Read the model definition and answer for the solid it produces. Units are mm, in the model's axes. Round coordinates to 2 decimals unless told otherwise and drop trailing zeros. Write each loop counter-clockwise with the first axis right and the second up, starting at its lowest first coordinate (ties: lowest second). Pieces come first, ordered by that corner, then holes.
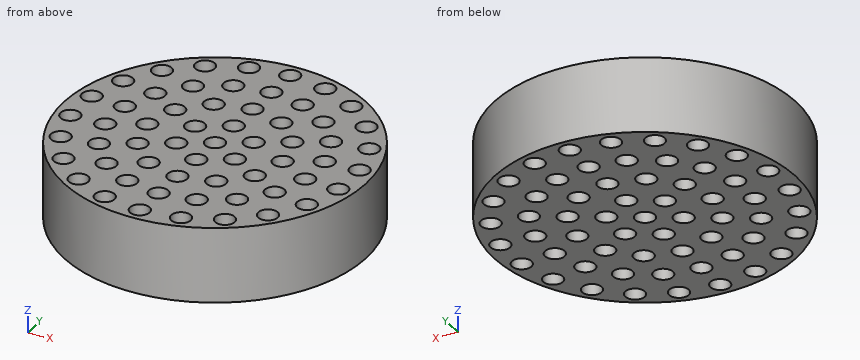
from build123d import *

# Parameters (mm, degrees)
ESQUISSE1_R             = 20
BOSS_EXTRU_1_DEPTH      = 10
ESQUISSE2_R             = 1.3
ENL_V_MAT_EXTRU_1_DEPTH = 10


with BuildPart() as part:
    # Esquisse1 → Boss.-Extru.1 (new body)
    with BuildSketch(Plane.XY):
        Circle(ESQUISSE1_R)
    extrude(amount=BOSS_EXTRU_1_DEPTH)

    # Esquisse2 → Enlèv. mat.-Extru.1 (cut)
    with BuildSketch(Plane.XY.offset(10)):
        with Locations((0, 4.5)):
            Circle(ESQUISSE2_R)
        with Locations((-3.897114317, 2.25)):
            Circle(ESQUISSE2_R)
        with Locations((-3.897114317, -2.25)):
            Circle(ESQUISSE2_R)
        with Locations((0, -4.5)):
            Circle(ESQUISSE2_R)
        with Locations((3.897114317, -2.25)):
            Circle(ESQUISSE2_R)
        with Locations((3.897114317, 2.25)):
            Circle(ESQUISSE2_R)
        Circle(ESQUISSE2_R)
        with Locations((0, 9)):
            Circle(ESQUISSE2_R)
        with Locations((4.5, 7.794228634)):
            Circle(ESQUISSE2_R)
        with Locations((7.794228634, 4.5)):
            Circle(ESQUISSE2_R)
        with Locations((9, 0)):
            Circle(ESQUISSE2_R)
        with Locations((7.794228634, -4.5)):
            Circle(ESQUISSE2_R)
        with Locations((4.5, -7.794228634)):
            Circle(ESQUISSE2_R)
        with Locations((0, -9)):
            Circle(ESQUISSE2_R)
        with Locations((-4.5, -7.794228634)):
            Circle(ESQUISSE2_R)
        with Locations((-7.794228634, -4.5)):
            Circle(ESQUISSE2_R)
        with Locations((-9, 0)):
            Circle(ESQUISSE2_R)
        with Locations((-7.794228634, 4.5)):
            Circle(ESQUISSE2_R)
        with Locations((-4.5, 7.794228634)):
            Circle(ESQUISSE2_R)
        with Locations((0, 13.5)):
            Circle(ESQUISSE2_R)
        with Locations((0, 18)):
            Circle(ESQUISSE2_R)
        with Locations((4.617271935, 12.685850381)):
            Circle(ESQUISSE2_R)
        with Locations((8.677632731, 10.341599982)):
            Circle(ESQUISSE2_R)
        with Locations((11.691342951, 6.75)):
            Circle(ESQUISSE2_R)
        with Locations((13.294904666, 2.344250399)):
            Circle(ESQUISSE2_R)
        with Locations((13.294904666, -2.344250399)):
            Circle(ESQUISSE2_R)
        with Locations((11.691342951, -6.75)):
            Circle(ESQUISSE2_R)
        with Locations((8.677632731, -10.341599982)):
            Circle(ESQUISSE2_R)
        with Locations((4.617271935, -12.685850381)):
            Circle(ESQUISSE2_R)
        with Locations((0, -13.5)):
            Circle(ESQUISSE2_R)
        with Locations((-4.617271935, -12.685850381)):
            Circle(ESQUISSE2_R)
        with Locations((-8.677632731, -10.341599982)):
            Circle(ESQUISSE2_R)
        with Locations((-11.691342951, -6.75)):
            Circle(ESQUISSE2_R)
        with Locations((-13.294904666, -2.344250399)):
            Circle(ESQUISSE2_R)
        with Locations((-13.294904666, 2.344250399)):
            Circle(ESQUISSE2_R)
        with Locations((-11.691342951, 6.75)):
            Circle(ESQUISSE2_R)
        with Locations((-8.677632731, 10.341599982)):
            Circle(ESQUISSE2_R)
        with Locations((-4.617271935, 12.685850381)):
            Circle(ESQUISSE2_R)
        with Locations((5.071186023, 17.270873525)):
            Circle(ESQUISSE2_R)
        with Locations((9.731534714, 15.142563591)):
            Circle(ESQUISSE2_R)
        with Locations((13.603492338, 11.787493211)):
            Circle(ESQUISSE2_R)
        with Locations((16.373375916, 7.477470234)):
            Circle(ESQUISSE2_R)
        with Locations((17.816785954, 2.561667089)):
            Circle(ESQUISSE2_R)
        with Locations((17.816785954, -2.561667089)):
            Circle(ESQUISSE2_R)
        with Locations((16.373375916, -7.477470234)):
            Circle(ESQUISSE2_R)
        with Locations((13.603492338, -11.787493211)):
            Circle(ESQUISSE2_R)
        with Locations((9.731534714, -15.142563591)):
            Circle(ESQUISSE2_R)
        with Locations((5.071186023, -17.270873525)):
            Circle(ESQUISSE2_R)
        with Locations((0, -18)):
            Circle(ESQUISSE2_R)
        with Locations((-5.071186023, -17.270873525)):
            Circle(ESQUISSE2_R)
        with Locations((-9.731534714, -15.142563591)):
            Circle(ESQUISSE2_R)
        with Locations((-13.603492338, -11.787493211)):
            Circle(ESQUISSE2_R)
        with Locations((-16.373375916, -7.477470234)):
            Circle(ESQUISSE2_R)
        with Locations((-17.816785954, -2.561667089)):
            Circle(ESQUISSE2_R)
        with Locations((-17.816785954, 2.561667089)):
            Circle(ESQUISSE2_R)
        with Locations((-16.373375916, 7.477470234)):
            Circle(ESQUISSE2_R)
        with Locations((-13.603492338, 11.787493211)):
            Circle(ESQUISSE2_R)
        with Locations((-9.731534714, 15.142563591)):
            Circle(ESQUISSE2_R)
        with Locations((-5.071186023, 17.270873525)):
            Circle(ESQUISSE2_R)
    extrude(amount=-ENL_V_MAT_EXTRU_1_DEPTH, mode=Mode.SUBTRACT)


solid = part.part
Q1. Section C-C (y = -18) is taken. Determine the outline of the cut face in (x, z).
Verdict:
outline: (-8.72, 0) - (-6.15, 0) - (-6.15, 10) - (-8.72, 10) - close; (-3.99, 0) - (-1.3, 0) - (-1.3, 10) - (-3.99, 10) - close; (1.3, 0) - (3.99, 0) - (3.99, 10) - (1.3, 10) - close; (6.15, 0) - (8.72, 0) - (8.72, 10) - (6.15, 10) - close
Q2. Flat-ended cylindrical pins translate along their axes: pin 1 Ø2 at (x, z) = (-2.5, 4.5) entering from +Y; pin 2 Ø1.6 at (x, y) = (9.73, 15.14) entering from +Z; pin 3 Ø6 at (x, z) = (-2, 1.5) entering from -Y; pin 4 Ø2 at (x, z) = (7.5, 9) entering from +Y. Find the tip coordinate at first contact, or state that the pin passes through.
Verdict:
pin 1: stops at y = 19.94
pin 2: passes through
pin 3: stops at y = -20
pin 4: stops at y = 18.91
Q3. Section A-A (y = -4.5) is taken. Determine the outline of the cut face in (x, z), then the cut area to 3 significant figures.
Verdict:
outline: (-19.49, 0) - (-9.09, 0) - (-9.09, 10) - (-19.49, 10) - close; (-6.49, 0) - (-1.3, 0) - (-1.3, 10) - (-6.49, 10) - close; (1.3, 0) - (6.49, 0) - (6.49, 10) - (1.3, 10) - close; (9.09, 0) - (19.49, 0) - (19.49, 10) - (9.09, 10) - close
area: 312 mm2
Q4. Straight lines are drawn through the part: probe 1 along X at (y, z) = (-11, 5); probe 2 along Y at (x, z) = (8, 3.5); probe 3 along X at (y, z) = (15, 1.75). For each, find the intervals that lie inside material, in ascending order.
Verdict:
probe 1: x = -16.7 to -14.64, -12.57 to -9.8, -7.56 to 7.56, 9.8 to 12.57, 14.64 to 16.7
probe 2: y = -18.33 to -11.45, -9.23 to -5.78, -3.22 to -0.83, 0.83 to 3.22, 5.78 to 9.23, 11.45 to 18.33
probe 3: x = -13.23 to -11.02, -8.44 to 8.44, 11.02 to 13.23
Q5. Section B-B (z = 6.75) is taken. State how many separate pieces and enclosed holes the cut face has, then the cut area to 3 significant figures.
Verdict:
separate pieces: 1
enclosed holes: 59
area: 943 mm2
